Autodesk Inventor part; units mm, degrees
ref_plane "YZ Plane" through (0, 0, 0) normal (1, 0, 0) x (0, 1, 0)
ref_plane "XZ Plane" through (0, 0, 0) normal (0, 1, 0) x (-1, 0, 0)
ref_plane "XY Plane" through (0, 0, 0) normal (0, 0, 1) x (1, 0, 0)
sketch "Sketch1" plane through (0, 0, 0) normal (0, 0, 1) x (1, 0, 0)
  line L0 (250, 9.5) -> (-250, 9.5)
  line L1 (-250, 9.5) -> (-250, -9.5)
  line L2 (-250, -9.5) -> (250, -9.5)
  line L3 (250, -9.5) -> (250, 9.5)
  line L4 (250, 9.5) -> (-250, -9.5) construction
  line L5 (-250, 9.5) -> (250, -9.5) construction
  point P0 (0, 0)
  dimension "d0" = 500
  dimension "d1" = 19
extrude "Extrusion1" add sketch "Sketch1" along normal blind 15
sketch "Sketch2" plane through (-250, 9.5, 0) normal (0, 1, 0) x (1, 0, 0)
  line L0 (0, 0) -> (0, -15)
  line L1 (0, 0) -> (15, -15)
  line L2 (0, -15) -> (500, -15)
  line L3 (0, 0) -> (0, -15)
  line L4 (15, -15) -> (0, -15)
  point P0 (250, 0)
  dimension "d5" = 45
extrude "Extrusion2" cut sketch "Sketch2" against normal through all
mirror "Mirror1" about plane through (0, 0, 0) normal (1, 0, 0) of "Extrusion2"
ref_plane "Work Plane1" through (0, 0, 0) normal (1, 0, 0) x (0, 1, 0)
properties part number "widthBinding"
Geometry: final body of the model. Coordinates: model frame, mm. Give positions to 0.01 mm unless a question says otherwise; leave off trailing zeros. Write each loop counter-clockwise with the first axis right and the second up, starting at its lowest first coordinate (ties: lowest second). Pieces come first, ordered by that corner, then holes.
1. Line query: probe 1 along X at (y, z) = (-6.5, 2.5); probe 2 along X at (y, z) = (-4.75, 10). Output: solid intervals per line, ascending.
2. Section query A-A, the plane y = 6.5. Return loops of the section in (x, z), then the cut area to 4 significant figures.
3. Section query B-B, the plane z = 6. Return loops of the section in (x, y).
4. Pin query (flat end, axial travel): P1, Ø1, axis at y = -1.5, z = 12.5, coming from the +X side; P2, Ø5, axis at y = -1, z = 12, coming from the -X side; P3, Ø4, axis at y = -4, z = 6, coming from the +X side. Return the tip coordinate at first contact, or that it passes through.
Computed:
1. probe 1: x = -247.5 to 247.5
1. probe 2: x = -240 to 240
2. outline: (-250, 0) - (250, 0) - (235, 15) - (-235, 15) - close
2. area: 7,275 mm2
3. outline: (-244, -9.5) - (244, -9.5) - (244, 9.5) - (-244, 9.5) - close
4. P1: stops at x = 238
4. P2: stops at x = -240.5
4. P3: stops at x = 246
